from build123d import *

# Parameters (mm, degrees)
SKETCH1_W           = 50
SKETCH1_H           = 50
SKETCH1_W_2         = 46
SKETCH1_H_2         = 46
BOSS_EXTRUDE1_DEPTH = 240
SKETCH2_W           = 46
SKETCH2_H           = 50
CUT_EXTRUDE1_DEPTH  = 247.424430607
CUT_EXTRUDE2_REACH  = 248.424
SKETCH3_R           = 6.5
SKETCH3_R_2         = 5
CUT_EXTRUDE3_REACH  = 248.424
SKETCH4_R           = 3
SKETCH4_R_2         = 5
SKETCH5_W           = 120
SKETCH5_H           = 46
CUT_EXTRUDE5_DEPTH  = 48
SKETCH6_R           = 2
CUT_EXTRUDE6_DEPTH  = 247.424430607


with BuildPart() as part:
    # Sketch1 → Boss-Extrude1 (new body)
    with BuildSketch(Plane.XY):
        Rectangle(SKETCH1_W, SKETCH1_H)
        Rectangle(SKETCH1_W_2, SKETCH1_H_2, mode=Mode.SUBTRACT)
    extrude(amount=-BOSS_EXTRUDE1_DEPTH)

    # Sketch2 → Cut-Extrude1 (cut, through all)
    with BuildSketch(Plane(origin=(0, 25, 0), x_dir=(1, 0, 0), z_dir=(0, 1, 0))):
        with Locations((0, 215)):
            Rectangle(SKETCH2_W, SKETCH2_H)
    extrude(amount=-CUT_EXTRUDE1_DEPTH, mode=Mode.SUBTRACT)

    # Sketch3 → Cut-Extrude2 (cut, up to next)
    with BuildSketch(Plane(origin=(25, 0, 0), x_dir=(0, 0, -1), z_dir=(1, 0, 0)), mode=Mode.PRIVATE) as cut_extrude2_sk1:
        with Locations((215, 0)):
            Circle(SKETCH3_R)
    cut_extrude2_tool1 = extrude(cut_extrude2_sk1.sketch, amount=-CUT_EXTRUDE2_REACH, mode=Mode.PRIVATE) & part.part
    # Sketch3 → Cut-Extrude2 (cut, up to next)
    with BuildSketch(Plane(origin=(25, 0, 0), x_dir=(0, 0, -1), z_dir=(1, 0, 0)), mode=Mode.PRIVATE) as cut_extrude2_sk2:
        with Locations((20, 0)):
            Circle(SKETCH3_R_2)
    cut_extrude2_tool2 = extrude(cut_extrude2_sk2.sketch, amount=-CUT_EXTRUDE2_REACH, mode=Mode.PRIVATE) & part.part
    add(cut_extrude2_tool1.solids().sort_by_distance((25, 0, -215))[0], mode=Mode.SUBTRACT)
    add(cut_extrude2_tool2.solids().sort_by_distance((25, 0, -20))[0], mode=Mode.SUBTRACT)

    # Sketch4 → Cut-Extrude3 (cut, up to next)
    with BuildSketch(Plane.ZY.offset(25), mode=Mode.PRIVATE) as cut_extrude3_sk1:
        with Locations((-215, 0)):
            Circle(SKETCH4_R)
    cut_extrude3_tool1 = extrude(cut_extrude3_sk1.sketch, amount=-CUT_EXTRUDE3_REACH, mode=Mode.PRIVATE) & part.part
    # Sketch4 → Cut-Extrude3 (cut, up to next)
    with BuildSketch(Plane.ZY.offset(25), mode=Mode.PRIVATE) as cut_extrude3_sk2:
        with Locations(Location((-20, 0, 0), (0, 0, 180))):
            Circle(SKETCH4_R_2)
    cut_extrude3_tool2 = extrude(cut_extrude3_sk2.sketch, amount=-CUT_EXTRUDE3_REACH, mode=Mode.PRIVATE) & part.part
    add(cut_extrude3_tool1.solids().sort_by_distance((-25, 0, -215))[0], mode=Mode.SUBTRACT)
    add(cut_extrude3_tool2.solids().sort_by_distance((-25, 0, -20))[0], mode=Mode.SUBTRACT)

    # Sketch5 → Cut-Extrude5 (cut)
    with BuildSketch(Plane(origin=(-25, 0, 0), x_dir=(0, 0, -1), z_dir=(1, 0, 0))):
        with Locations((115, 0)):
            Rectangle(SKETCH5_W, SKETCH5_H)
    extrude(amount=CUT_EXTRUDE5_DEPTH, mode=Mode.SUBTRACT)

    # Sketch6 → Cut-Extrude6 (cut, through all)
    with BuildSketch(Plane(origin=(0, 25, 0), x_dir=(1, 0, 0), z_dir=(0, 1, 0))):
        with Locations(Location((0, 20, 0), (0, 0, 270))):
            Circle(SKETCH6_R)
    extrude(amount=-CUT_EXTRUDE6_DEPTH, mode=Mode.SUBTRACT)


solid = part.part
The model under review builds one solid part; all positions refer to its coordinate system, in mm. A direction names the side the tool comes from. Coordinates: 2 decimals unless noted, no trailing zeros. Loops run counter-clockwise (first coordinate to the right, second up) from the corner with the lowest first, then second, coordinate; pieces in that order, holes last. Notation, with made-up numbers: M 77.5,34.5 L 95.5,34.5 A24 ccw 95.5,55.5 Z; hole C -25.75,49 d10. An arc over 180 degrees is marked long. Put each result on its own line as item: value. Start each with the question number.
Q1. Add section B-B (y = 18). Write out the cut boundary in (x, z), and give its area (3 significant figures).
Q2. Wall thickness on line 1 (Y direction, x = 23.9, z = -215); line 2 (Y direction, x = 1, z = -17.5): over which ranges is each line inside the solid? List them lowest first.
Q3. For faces 5 (the flat face through (-25, 0, -38)), 6 (the flat face through (-23, 0, -27)), 7 (the cylindrical face through (24.014, 0.286, -208.506)), list the 3-axis set-ups (+Z, -Z, +X, -X, +Y, -Y) from which the entire face can be reached by the end or side of a thin tool; tool diameter is ignored.
Q4. Add section C-C (x = 6.5). Write out the cut boundary in (y, z), and give its area (3 significant figures).
Q5. The part is to be moulded in two halves that separate along Y. For faces 1 (the flat face through (-2, -24, 0)), 2 (the flat face through (-23, 0, -207)), 3 (the cylindrical face through (-24, 0, -15)), 4 (the flat face through (0, -25, -92)), say which applies: +Y half, -Y half, draft (parallel to the pull), parting line (faces both ways), or undercut.
Q6. Clearance check with flat-ended pins moving along their axes: pin 1 (3 mm diameter, centred on y = -8, z = -123.5, fed in from -X); pin 2 (3.5 mm diameter, centred on x = 0, z = -20, fed in from -Y); pin 3 (11.5 mm diameter, centred on y = 0, z = -20, fed in from +X); pin 4 (10.5 mm diameter, centred on y = 0, z = -215, fed in from +X). State where each tip first meets the part, or that it passes through.
Q7. Add section D-D (y = 0). Write out the cut boundary in (x, z).
Q8. Add section A-A (z = -215). Write out the cut boundary in (x, y).
Answers:
1. outline: M -25,-240 L -23,-240 L -23,-175 L -25,-175 Z; M -25,-55 L -23,-55 L -23,0 L -25,0 Z; M 23,-240 L 25,-240 L 25,0 L 23,0 Z
1. area: 720 mm^2
2. line 1: y = -25 to -6.5, 6.5 to 25
2. line 2: y = -25 to -23, 23 to 25
3. face 5: +Z, -Z, -X, +Y, -Y
3. face 6: +Z, -Z
3. face 7: +X
4. outline: M -25,-190 L -23,-190 L -23,0 L -25,0 Z; M 23,-190 L 25,-190 L 25,0 L 23,0 Z
4. area: 760 mm^2
5. face 1: draft
5. face 2: undercut
5. face 3: undercut
5. face 4: -Y half
6. pin 1: stops at x = 23
6. pin 2: passes through
6. pin 3: stops at x = 25
6. pin 4: stops at x = -23
7. outline: M -25,-240 L -23,-240 L -23,-218 L -25,-218 Z; M -25,-212 L -23,-212 L -23,-175 L -25,-175 Z; M -25,-55 L -23,-55 L -23,-25 L -25,-25 Z; M -25,-15 L -23,-15 L -23,0 L -25,0 Z; M 23,-240 L 25,-240 L 25,-221.5 L 23,-221.5 Z; M 23,-208.5 L 25,-208.5 L 25,-25 L 23,-25 Z; M 23,-15 L 25,-15 L 25,0 L 23,0 Z
8. outline: M -25,-25 L -23,-25 L -23,-3 L -25,-3 Z; M -25,3 L -23,3 L -23,25 L -25,25 Z; M 23,-25 L 25,-25 L 25,-6.5 L 23,-6.5 Z; M 23,6.5 L 25,6.5 L 25,25 L 23,25 Z
